Check sheet for the modelled part. Datum: model origin and axes. Units: mm. A direction names the side the tool comes from. Give positions to 0.01 mm unless a question says otherwise; leave off trailing zeros. Write each loop counter-clockwise with the first axis right and the second up, starting at its lowest first coordinate (ties: lowest second). Pieces come first, ordered by that corner, then holes. Notation, with made-up numbers: M 88,0.25 L 98,0.25 A18 cw 98,34.25 Z; hole C 70.5,-15 d4. An arc over 180 degrees is marked long. Write item = value, one per line. Start each with the question number.
1) Cross-section at D-D, the plane y = -42. Record the cut outline in (x, z), plus the area to 3 significant figures.
2) Cross-section at B-B, the plane x = 26.5. Record the cut outline in (y, z).
3) Access from +Z, -Z, +X, -X, +Y, -Y to the whole of each face (thin tool, end or side, straight path). Record for faces 1 (the flat face through (22, -25, 3)), 2 (the cylindrical face through (1.5, -28, 26.6)).
4) Scan lines: line 1 along Z through (x, y) = (2, -25); line 2 along Z through (x, y) = (46.5, -27.5). Record each from-to range of solid material in increasing order. Write a range as [from, to].
5) Mould release check, pull along X, two halves, no side actions. Record for faces 3 (the flat face through (50, -25, 1)), 4 (the flat face through (2, -25, 50)), 5 (the cylindrical face through (23.5, -24.9, 1.5)): released by +X, released by -X, zero draft, split by the parting line, or undercut.
6) Cross-section at A-A, the plane y = -25. Record the cut outline in (x, z).
7) Go/stop test with flat-tipped pins: pin 1 (23.5 mm diameter, centred on y = -29, z = 18.5, fed in from +X); pin 2 (3 mm diameter, centred on x = 33, y = -32.5, fed in from +Z); pin 3 (5 mm diameter, centred on y = -15, z = 15.5, fed in from -X). Record where each tip stops, or that it passes through.
8) Cross-section at C-C, the plane z = 26.5. Record the cut outline in (x, y).
```python
from build123d import *

# Parameters (mm, degrees)
F1_DEPTH = 50
F2_R     = 3
F3_DEPTH = 3
F4_R     = 3
F5_DEPTH = 3.001


with BuildPart() as f1:
    # F0 (on Front) → F1 (new body)
    with BuildSketch(Plane.XZ):
        Polygon((0, 50), (0, 0), (50, 0), (50, 3), (3, 3), (3, 50), align=None)
    extrude(amount=F1_DEPTH)

    # F2 (on face) → F3 (cut, through all)
    with BuildSketch(Plane.YZ.offset(3)):
        with Locations((-25, 26.5)):
            Circle(F2_R)
    extrude(amount=-F3_DEPTH, mode=Mode.SUBTRACT)

    # F4 (on face) → F5 (cut, through all)
    with BuildSketch(Plane.XY.offset(3)):
        with Locations((26.5, -25)):
            Circle(F4_R)
    extrude(amount=-F5_DEPTH, mode=Mode.SUBTRACT)


solid = f1.part
```
Reply:
q1.outline = M 0,0 L 50,0 L 50,3 L 3,3 L 3,50 L 0,50 Z
q1.area = 291 mm2
q2.outline = M -50,0 L -28,0 L -28,3 L -50,3 Z; M -22,0 L 0,0 L 0,3 L -22,3 Z
q3.face_1 = +Z, +X, +Y, -Y
q3.face_2 = +X, -X
q4.line_1 = [0, 23.5], [29.5, 50]
q4.line_2 = [0, 3]
q5.face_3 = released by +X
q5.face_4 = zero draft
q5.face_5 = undercut
q6.outline = M 0,0 L 23.5,0 L 23.5,3 L 3,3 L 3,23.5 L 0,23.5 Z; M 0,29.5 L 3,29.5 L 3,50 L 0,50 Z; M 29.5,0 L 50,0 L 50,3 L 29.5,3 Z
q7.pin_1 = 3
q7.pin_2 = 3
q7.pin_3 = 0
q8.outline = M 0,-50 L 3,-50 L 3,-28 L 0,-28 Z; M 0,-22 L 3,-22 L 3,0 L 0,0 Z
